Autodesk Inventor part; units mm, degrees
ref_plane "YZ Plane" through (0, 0, 0) normal (1, 0, 0) x (0, 1, 0)
ref_plane "XZ Plane" through (0, 0, 0) normal (0, 1, 0) x (-1, 0, 0)
ref_plane "XY Plane" through (0, 0, 0) normal (0, 0, 1) x (1, 0, 0)
sketch "Esquisse1" plane through (0, 0, 0) normal (0, 0, 1) x (1, 0, 0)
  line L0 (0, 0) -> (34.4, 0)
  line L1 (34.4, 0) -> (34.4, 20)
  line L2 (34.4, 20) -> (0, 20)
  line L3 (0, 20) -> (0, 0)
  dimension "d0" = 34.4
  dimension "d1" = 20
extrude "Extrusion1" add sketch "Esquisse1" along normal blind 2.2
sketch "Esquisse2" plane through (0, 0, 2.2) normal (0, 0, 1) x (1, 0, 0)
  line L0 (0, 0) -> (34.4, 0)
  line L1 (34.4, 20) -> (0, 20)
  line L2 (0, 20) -> (0, 0)
  line L3 (0, 20) -> (2.2, 20)
  line L4 (2.2, 20) -> (2.2, 0)
  line L5 (2.2, 0) -> (0, 0)
  line L6 (0, 0) -> (0, 20)
  line L7 (17.2, 20) -> (17.2, 0) construction
  line L8 (34.4, 20) -> (32.2, 20)
  line L9 (32.2, 20) -> (32.2, 0)
  line L10 (32.2, 0) -> (34.4, 0)
  line L11 (34.4, 0) -> (34.4, 20)
  dimension "d4" = 2.2
extrude "Extrusion2" add sketch "Esquisse2" along normal blind 27 contours L2 L1 L4 L0 | L9 L1 L11 L0
sketch "Esquisse3" plane through (34.4, 0, 0) normal (1, 0, 0) x (0, 0, -1)
  line L0 (0, 0) -> (0, 20) construction
  line L1 (-29.2, 0) -> (-29.2, 20) construction
  line L2 (-29.2, 10) -> (0, 10) construction
  circle A0 centre (-20.2, 10) radius 2.15
  line L3 (-20.2, 10) -> (-20.2, 15.2246) construction
  circle A1 centre (-14.2, 10) radius 2.15
  circle A2 centre (-26.2, 10) radius 2.15
  circle A3 centre (-20.2, 10) radius 2.15
  circle A4 centre (-20.2, 16) radius 2.15
  circle A5 centre (-20.2, 4) radius 2.15
  circle A6 centre (-20.2, 10) radius 2.15
  dimension "d7" = 9
  dimension "d8" = 4.3
  dimension "d11" = 6
  dimension "d14" = 6
  dimension "d19" = 6
  dimension "d22" = 6
extrude "Extrusion3" cut sketch "Esquisse3" against normal through all
fillet "Congé1" radius 8 4 edges at (33.3, 20, 29.2) (1.1, 20, 29.2) (1.1, 0, 29.2) (33.3, 0, 29.2)
fillet "Congé2" radius 8 4 edges at (2.2, 10, 2.2) (0, 10, 0) (34.4, 10, 0) (32.2, 10, 2.2)
sketch "Esquisse4" plane through (0, 0, 0) normal (0, 0, -1) x (-1, 0, 0)
  line L0 (-8, 0) -> (-26.4, 0) construction
  line L1 (-26.4, 20) -> (-8.3748, 0) construction
  line L2 (-23.3874, 4) -> (-11.3874, 4) construction
  line L3 (-11.3874, 4) -> (-11.3874, 16) construction
  line L4 (-11.3874, 16) -> (-23.3874, 16) construction
  line L5 (-23.3874, 16) -> (-23.3874, 4) construction
  line L6 (-23.3874, 4) -> (-11.3874, 16) construction
  line L7 (-11.3874, 4) -> (-23.3874, 16) construction
  circle A0 centre (-23.3874, 16) radius 1.25
  line L8 (-17.3874, 16) -> (-17.3874, 4) construction
  line L9 (-23.3874, 10) -> (-11.3874, 10) construction
  circle A1 centre (-11.3874, 16) radius 1.25
  circle A2 centre (-23.3874, 4) radius 1.25
  circle A3 centre (-11.3874, 4) radius 1.25
  point P0 (0, 0)
  point P1 (-17.3874, 10)
  dimension "d29" = 12
  dimension "d30" = 2.5
extrude "Extrusion4" cut sketch "Esquisse4" against normal through all
equation "\"d2\" = UDepth"
equation "\"d4\" = Depth"
equation "\"d8\" = Holes"
equation "\"d28\" = URound"
equation "\"Depth\" = 2.2"
equation "\"Holes\" = 4.3"
equation "\"UDepth\" = Depth"
equation "\"USize\" = 5"
equation "\"URound\" = 8"
properties part number "Ufix"
Geometry check sheet. Reference: the model listing, model coordinates, mm. A direction names the side the tool comes from. Round coordinates to 2 decimals unless told otherwise and drop trailing zeros. Order: outer loops, then holes, each group sorted by start corner. A loop starts at its lowest first (then second) coordinate and runs counter-clockwise, first axis right, second up. Notation, with made-up numbers: (-7, 49.25) -> (8, 49.25) arc R4 ccw to (8, 56.25) -> close; hole circle Ø7 at (52, -16). An arc over 180 degrees is marked (long way). Return JSON: item names as keys, results as strings. Group by question number.
Q1. Section check C-C, the plane z = 7. Record the boundary of the cut face in (x, y), plus the area to 3 significant figures.
Q2. Tool access check on faces 1 (the cylindrical face through (24.636, 16.055, 1.091)), 2 (the flat face through (32.2, 10, 17)). Record the directions out of +Z, -Z, +X, -X, +Y, -Y that give a thin tool (end or side, any length) a straight path to the whole face; none if there is none.
Q3. Section check D-D, the plane x = 19.5. Record the boundary of the cut face in (y, z), plus the area to 3 significant figures.
Q4. Section check B-B, the plane z = 14.25. Record the boundary of the cut face in (x, y).
Q5. Release check for a two-part mould opening along Z. For faces 3 (the cylindrical face through (1.085, 17.594, 26.919)), 4 (the cylindrical face through (33.32, 10.09, 16.35)), 5 (the flat face through (34.4, 8, 18)) record: released by +Z, released by -Z, zero draft, split by the parting line, or undercut.
Q6. Section check A-A, the plane z = 20.2. Count the separate pieces of the cut face and the enclosed holes in it, plus the area to 3 significant figures.
Q7. Gauge pin test, flat ends, axial feed: pin 1 (10 mm diameter, centred on x = 28.5, y = 15, fed in from -Z); pin 2 (4 mm diameter, centred on x = 19, y = 14.5, fed in from +Z); pin 3 (4 mm diameter, centred on x = 23.39, y = 16, fed in from +Z); pin 4 (5 mm diameter, centred on y = 18, z = 3.5, fed in from +X). Record the tip position at first contact, or that the pin passes through.
Q8. Material ranges on probe 1 along Y at (x, z) = (33.4, 20.2); probe 2 along X at (y, z) = (6.25, 17.25); probe 3 along Y at (x, z) = (1.35, 14.2), recorded low to high. Write a range as from..to.
Numbers:
{
 "1": {"outline": "(0.06, 0) -> (2.87, 0) -> (2.87, 20) -> (0.06, 20) -> close; (31.53, 0) -> (34.34, 0) -> (34.34, 20) -> (31.53, 20) -> close", "area": "112 mm^2"},
 "2": {"face 1": "+Z, -Z", "face 2": "+Z, +Y, -Y"},
 "3": {"outline": "(0, 0) -> (20, 0) -> (20, 2.2) -> (0, 2.2) -> close", "area": "44.0 mm^2"},
 "4": {"outline": "(0, 0) -> (2.2, 0) -> (2.2, 7.85) -> (0, 7.85) -> close; (0, 12.15) -> (2.2, 12.15) -> (2.2, 20) -> (0, 20) -> close; (32.2, 0) -> (34.4, 0) -> (34.4, 7.85) -> (32.2, 7.85) -> close; (32.2, 12.15) -> (34.4, 12.15) -> (34.4, 20) -> (32.2, 20) -> close"},
 "5": {"face 3": "released by +Z", "face 4": "undercut", "face 5": "zero draft"},
 "6": {"separate pieces": "8", "enclosed holes": "0", "area": "31.2 mm^2"},
 "7": {"pin 1": "z = 0", "pin 2": "z = 2.2", "pin 3": "z = 2.29", "pin 4": "x = 34.15"},
 "8": {"probe 1": "0..1.85, 6.15..7.85, 12.15..13.85, 18.15..20", "probe 2": "0..2.2, 32.2..34.4", "probe 3": "0..7.85, 12.15..20"}
}
